Input: part model. Units: mm. Frame: model coordinates. A direction names the side the tool comes from. Round coordinates to 2 decimals unless told otherwise and drop trailing zeros. Loops run counter-clockwise (first coordinate to the right, second up) from the corner with the lowest first, then second, coordinate; pieces in that order, holes last. Notation, with made-up numbers: (-1, 15) -> (31, 15) arc R19 ccw to (31, 50) -> close; hole circle Ø7 at (44, 21). An arc over 180 degrees is marked (long way). Answer in a Markdown table with one row per item. Add a question column.
Q1. Reachability of faces 1 (the face through (4.762, 15, 26)), 2 (the face through (7, 12.7, 11)), 3 (the face through (4.762, 15, -26)) from +Z, -Z, +X, -X, +Y, -Y: full face, straight path, thin tool, end or side. Return the list, or none.
Q2. Pin query (flat end, axial travel): pin 1 (4 mm diameter, centred on x = -8.5, y = -9.5, fed in from +Z); pin 2 (2 mm diameter, centred on y = 7, z = -3, fed in from +X); pin 3 (8 mm diameter, centred on x = -12, y = -1, fed in from +Z). Return the tip coordinate at first contact, or that it passes through.
Q3. Section B-B, the plane x = 0. Give the number of separate pieces and of enclosed holes in the cut face, and give its area (3 significant figures).
Q4. Section A-A, the plane z = 32.5. Output: boundary loops of the cut face in (x, y).
Q5. Section C-C, the plane x = 4. Output: boundary loops of the cut face in (y, z), and give its area (3 significant figures).
Q6. Ray query, L1, parallel to Z at x = 0, y = 16.35 (3 decimals); L2, parallel to Y at x = -0.25, z = -27.5; L3, parallel to Z at x = 4, y = 15.5. Return the intervals inside material, ascending. Write a range as from..to.
Q7. Mould query, pull axis Z, two halves, no side actions, for faces 4 (the face through (0, 15, -37.5)), 5 (the face through (-0.067, 15.756, -27.07)), 6 (the face through (-15.873, 15.048, -0.281)). Classes: pulls with the +Z half, pulls with the -Z half, needs draft (parallel to the pull), parting line crosses it, or undercut.
Q8. Section D-D, the plane y = -1. Output: boundary loops of the cut face in (x, z) (3 decimals).
```python
from build123d import *

# Parameters (mm, degrees)
SKETCH2_R             = 12.7
SKETCH2_R_2           = 9.525
BOSS_EXTRUDE1_DEPTH   = 12.7
SKETCH3_R             = 12.7
BOSS_EXTRUDE2_DEPTH   = 4.7625
SKETCH4_R             = 9.525
CUT_EXTRUDE1_DEPTH    = 5.7625
M4_CLEARANCE_HOLE1_D  = 4.5
M2X0_4_TAPPED_HOLE1_D = 1.6


with BuildPart() as part:
    # Sketch2 → Boss-Extrude1 (new body, symmetric)
    with BuildSketch(Plane(origin=(0, 0, 0), x_dir=(1, 0, 0), z_dir=(0, 1, 0))):
        Circle(SKETCH2_R)
        Circle(SKETCH2_R_2, mode=Mode.SUBTRACT)
    extrude(amount=BOSS_EXTRUDE1_DEPTH, both=True)

    # Sketch3 → Boss-Extrude2 (add)
    with BuildSketch(Plane(origin=(0, 12.7, 0), x_dir=(1, 0, 0), z_dir=(0, 1, 0))):
        with BuildLine():
            ThreePointArc((-4.7625, -15.143784822), (0, -15.875), (4.7625, -15.143784822))
            Line((4.7625, -15.143784822), (4.7625, -11.773215098))
            ThreePointArc((4.7625, -11.773215098), (0, -12.7), (-4.7625, -11.773215098))
            Line((-4.7625, -11.773215098), (-4.7625, -15.143784822))
        make_face()
        with BuildLine():
            ThreePointArc((4.7625, 15.143784822), (0, 15.875), (-4.7625, 15.143784822))
            Line((-4.7625, 15.143784822), (-4.7625, 11.773215098))
            ThreePointArc((-4.7625, 11.773215098), (0, 12.7), (4.7625, 11.773215098))
            Line((4.7625, 11.773215098), (4.7625, 15.143784822))
        make_face()
        with BuildLine():
            Line((-4.7625, -37.5), (4.7625, -37.5))
            Line((4.7625, -37.5), (4.7625, -15.143784822))
            ThreePointArc((4.7625, -15.143784822), (0, -15.875), (-4.7625, -15.143784822))
            Line((-4.7625, -15.143784822), (-4.7625, -37.5))
        make_face()
        with BuildLine():
            Line((-4.7625, 37.5), (-4.7625, 15.143784822))
            ThreePointArc((-4.7625, 15.143784822), (0, 15.875), (4.7625, 15.143784822))
            Line((4.7625, 15.143784822), (4.7625, 37.5))
            Line((4.7625, 37.5), (-4.7625, 37.5))
        make_face()
        with BuildLine():
            Line((4.7625, -11.773215098), (4.7625, -15.143784822))
            ThreePointArc((4.7625, -15.143784822), (12.798834175, -9.391776656), (15.875, 0))
            ThreePointArc((15.875, 0), (12.798834175, 9.391776656), (4.7625, 15.143784822))
            Line((4.7625, 15.143784822), (4.7625, 11.773215098))
            ThreePointArc((4.7625, 11.773215098), (10.530283709, 7.099515829), (12.7, 0))
            ThreePointArc((12.7, 0), (10.530283709, -7.099515829), (4.7625, -11.773215098))
        make_face()
        with BuildLine():
            ThreePointArc((-4.7625, 15.143784822), (-15.875, 0), (-4.7625, -15.143784822))
            Line((-4.7625, -15.143784822), (-4.7625, -11.773215098))
            ThreePointArc((-4.7625, -11.773215098), (-12.7, 0), (-4.7625, 11.773215098))
            Line((-4.7625, 11.773215098), (-4.7625, 15.143784822))
        make_face()
        Circle(SKETCH3_R)
    extrude(amount=BOSS_EXTRUDE2_DEPTH)

    # Sketch4 → Cut-Extrude1 (cut, through all)
    with BuildSketch(Plane.XZ.offset(-12.7)):
        Circle(SKETCH4_R)
    extrude(amount=-CUT_EXTRUDE1_DEPTH, mode=Mode.SUBTRACT)

    # M4 Clearance Hole1 (through all)
    with Locations(Plane(origin=(0, 12.7, 0), x_dir=(-1, 0, 0), z_dir=(0, -1, 0))):
        with Locations((0, 32.5), (0, 22.5), (0, -22.5), (0, -32.5)):
            Hole(M4_CLEARANCE_HOLE1_D / 2)

    # M2x0.4 Tapped Hole1 (through all)
    with Locations(Plane(origin=(4.7625, 0, 0), x_dir=(0, 0, -1), z_dir=(1, 0, 0))):
        with Locations((27.5, 15.08125)):
            Hole(M2X0_4_TAPPED_HOLE1_D / 2)


solid = part.part
```
Answer block:
| question | item | result |
|---|---|---|
| 1 | face 1 | +Z, +X, +Y, -Y |
| 1 | face 2 | -Y |
| 1 | face 3 | -Z, +X, +Y, -Y |
| 2 | pin 1 | z = 10.91 |
| 2 | pin 2 | x = 12.54 |
| 2 | pin 3 | z = 9.86 |
| 3 | separate pieces | 6 |
| 3 | enclosed holes | 1 |
| 3 | area | 340 mm^2 |
| 4 | outline | (-4.76, 12.7) -> (-2.25, 12.7) -> (-2.25, 17.46) -> (-4.76, 17.46) -> close; (2.25, 12.7) -> (4.76, 12.7) -> (4.76, 17.46) -> (2.25, 17.46) -> close |
| 5 | outline | (-12.7, -12.05) -> (12.7, -12.05) -> (12.7, -37.5) -> (17.46, -37.5) -> (17.46, -8.64) -> (-12.7, -8.64) -> close; (-12.7, 8.64) -> (17.46, 8.64) -> (17.46, 37.5) -> (12.7, 37.5) -> (12.7, 12.05) -> (-12.7, 12.05) -> close; hole circle Ø1.6 at (15.08, -27.5) |
| 5 | area | 446 mm^2 |
| 6 | L1 | -37.5..-34.75, -30.25..-24.75, -20.25..-9.525, 9.525..20.25, 24.75..30.25, 34.75..37.5 |
| 6 | L2 | 12.7..14.28, 15.88..17.46 |
| 6 | L3 | -37.5..-28.18, -26.82..-8.64, 8.64..37.5 |
| 7 | face 4 | pulls with the -Z half |
| 7 | face 5 | undercut |
| 7 | face 6 | parting line crosses it |
| 8 | outline | circle Ø25.4 at (0, 0); hole circle Ø19.05 at (0, 0) |
